Source: CAD feature listing. Evaluate the final solid. Frame: model axes, mm. A direction names the side the tool comes from. Give positions to 0.01 mm unless a question says otherwise; leave off trailing zeros. Loops run counter-clockwise (first coordinate to the right, second up) from the corner with the lowest first, then second, coordinate; pieces in that order, holes last. Notation, with made-up numbers: (27.25, -25.5) - (57.25, -25.5) arc R33 ccw to (57.25, 2.5) - close; hole circle Ø6 at (39, 72). An arc over 180 degrees is marked (long way). Put each result on its own line as item: value.
```python
from build123d import *

# Parameters (mm, degrees)
SKETCH1_R            = 14.2875
SKETCH1_R_2          = 2.54
BOSS_EXTRUDE1_DEPTH  = 3.175
CUT_EXTRUDE1_DEPTH   = 162.674043733
FILLET3_R            = 6.35
BOSS_EXTRUDE3_START  = -3.175
SKETCH3_R            = 2.54
BOSS_EXTRUDE3_DEPTH  = 3.175
SKETCH6_R            = 2.54
BOSS_EXTRUDE4_DEPTH  = 3.175
FILLET2_R            = 6.35
CUT_EXTRUDE2_DEPTH   = 168.423732074
CUT_EXTRUDE3_DEPTH   = 168.423732074
CUT_EXTRUDE4_DEPTH   = 168.265702461
BOSS_EXTRUDE8_START  = -3.175
SKETCH15_R           = 2.54
BOSS_EXTRUDE8_DEPTH  = 3.175
FILLET4_R            = 2.54
BOSS_EXTRUDE9_DEPTH  = 3.175
SKETCH17_R           = 14.2875
BOSS_EXTRUDE10_DEPTH = 3.175
CUT_EXTRUDE5_DEPTH   = 132.939082706
SKETCH20_R           = 14.2875
CUT_EXTRUDE6_DEPTH   = 132.939082706


with BuildPart() as part:
    # Sketch1 → Boss-Extrude1 (new body)
    with BuildSketch(Plane.XY):
        with BuildLine():
            Line((-8.89, 25.4), (8.89, 25.4))
            ThreePointArc((8.89, 25.4), (17.870256121, 21.680256121), (21.59, 12.7))
            Line((21.59, 12.7), (21.59, -117.775079775))
            ThreePointArc((21.59, -117.775079775), (21.127743647, -120.388718212), (19.797058824, -122.685251408))
            Line((19.797058824, -122.685251408), (-7.952696208, -155.616779465))
            ThreePointArc((-7.952696208, -155.616779465), (-12.268297602, -157.851943494), (-16.900388255, -156.380852124))
            Line((-16.900388255, -156.380852124), (-32.439211784, -143.287061102))
            ThreePointArc((-32.439211784, -143.287061102), (-34.674375812, -138.971459708), (-33.203284443, -134.339369055))
            Line((-33.203284443, -134.339369055), (-23.382941176, -122.685251408))
            ThreePointArc((-23.382941176, -122.685251408), (-22.052256353, -120.388718212), (-21.59, -117.775079775))
            Line((-21.59, -117.775079775), (-21.59, 12.7))
            ThreePointArc((-21.59, 12.7), (-17.870256121, 21.680256121), (-8.89, 25.4))
        make_face()
        Circle(SKETCH1_R, mode=Mode.SUBTRACT)
        with Locations((0, -101.6)):
            Circle(SKETCH1_R, mode=Mode.SUBTRACT)
        with Locations((-18.532085478, -142.550133084)):
            Circle(SKETCH1_R_2, mode=Mode.SUBTRACT)
        with Locations((0, -50.8)):
            Circle(SKETCH1_R_2, mode=Mode.SUBTRACT)
    extrude(amount=BOSS_EXTRUDE1_DEPTH)

    # Sketch2 → Cut-Extrude1 (cut, through all)
    with BuildSketch(Plane.XY):
        with BuildLine():
            ThreePointArc((19.159083004, -91.647229609), (9.182340769, -50.8), (19.159083004, -9.952770391))
            ThreePointArc((19.159083004, -9.952770391), (20.973467787, -5.122670102), (21.59, 0))
            Line((21.59, 0), (27.94, 0))
            Line((27.94, 0), (27.94, -121.656687185))
            Line((27.94, -121.656687185), (-7.789552878, -164.05809836))
            Line((-7.789552878, -164.05809836), (-17.501317584, -155.874478972))
            Line((-17.501317584, -155.874478972), (16.51, -115.512152961))
            ThreePointArc((16.51, -115.512152961), (20.280273667, -109.005308906), (21.59, -101.6))
            ThreePointArc((21.59, -101.6), (20.973467787, -96.477329898), (19.159083004, -91.647229609))
        make_face()
        with BuildLine():
            Line((-21.59, -41.275), (-21.59, -60.325))
            ThreePointArc((-21.59, -60.325), (-12.065, -50.8), (-21.59, -41.275))
        make_face()
    extrude(amount=CUT_EXTRUDE1_DEPTH, mode=Mode.SUBTRACT)

    # Fillet3
    fillet3_edges = [part.edges().sort_by_distance(p)[0] for p in [
        (-21.59, -41.275, 1.5875),
        (-21.59, -60.325, 1.5875),
    ]]
    fillet(fillet3_edges, radius=FILLET3_R)

    # Sketch3 → Boss-Extrude3 (add)
    with BuildSketch(Plane.XY.offset(3.175).offset(BOSS_EXTRUDE3_START)):
        with BuildLine():
            Line((-27.351416194, -127.394768527), (-36.025496499, -137.688579))
            ThreePointArc((-36.025496499, -137.688579), (-37.217489152, -141.441859142), (-35.4063854, -144.93869507))
            Line((-35.4063854, -144.93869507), (-24.403104784, -154.210610454))
            ThreePointArc((-24.403104784, -154.210610454), (-19.771014132, -155.681701823), (-15.455412737, -153.446537795))
            Line((-15.455412737, -153.446537795), (-7.557639641, -144.073996091))
            Line((-7.557639641, -144.073996091), (-27.351416194, -127.394768527))
        make_face()
        with Locations((-18.532085478, -142.550133084)):
            Circle(SKETCH3_R, mode=Mode.SUBTRACT)
    extrude(amount=BOSS_EXTRUDE3_DEPTH)

    # Sketch6 → Boss-Extrude4 (add)
    with BuildSketch(Plane.XY.offset(3.175)):
        Polygon((-35.4063854, -144.93869507), (-63.620410749, -121.164144113), (-51.344981666, -106.596497054), (-27.065569901, -127.055545526), align=None)
        with Locations((-52.626813855, -117.972130278)):
            Circle(SKETCH6_R, mode=Mode.SUBTRACT)
    extrude(amount=-BOSS_EXTRUDE4_DEPTH)

    # Fillet2
    fillet2_edges = [part.edges().sort_by_distance(p)[0] for p in [
        (-63.620410749, -121.164144113, 1.5875),
        (-51.344981666, -106.596497054, 1.5875),
        (-27.065569901, -127.055545526, 1.5875),
    ]]
    fillet(fillet2_edges, radius=FILLET2_R)

    # Sketch7 → Cut-Extrude2 (cut, through all)
    with BuildSketch(Plane.XY.offset(3.175)):
        with BuildLine():
            Line((-21.59, 0), (-21.59, 31.75))
            Line((-21.59, 31.75), (21.59, 31.75))
            Line((21.59, 31.75), (21.59, 0))
            ThreePointArc((21.59, 0), (0, 21.59), (-21.59, 0))
        make_face()
    extrude(amount=-CUT_EXTRUDE2_DEPTH, mode=Mode.SUBTRACT)

    # Sketch10 → Cut-Extrude3 (cut, through all)
    with BuildSketch(Plane.XY.offset(3.175)):
        with BuildLine():
            Line((-18.151882461, -155.32628042), (-17.361482582, -157.512020269))
            Line((-17.361482582, -157.512020269), (-14.375706423, -156.432313955))
            Line((-14.375706423, -156.432313955), (-15.455412737, -153.446537795))
            ThreePointArc((-15.455412737, -153.446537795), (-16.679911193, -154.563907595), (-18.151882461, -155.32628042))
        make_face()
    extrude(amount=-CUT_EXTRUDE3_DEPTH, mode=Mode.SUBTRACT)

    # Sketch12 → Cut-Extrude4 (cut, through all)
    with BuildSketch(Plane.XY.offset(3.175)):
        with BuildLine():
            Line((-21.59, -101.6), (-72.39, -101.6))
            Line((-72.39, -101.6), (-72.39, -165.1))
            Line((-72.39, -165.1), (16.51, -165.1))
            Line((16.51, -165.1), (16.51, -115.512152961))
            ThreePointArc((16.51, -115.512152961), (-7.405308906, -121.880273667), (-21.59, -101.6))
        make_face()
    extrude(amount=-CUT_EXTRUDE4_DEPTH, mode=Mode.SUBTRACT)

    # Sketch15 → Boss-Extrude8 (add)
    with BuildSketch(Plane.XY.offset(3.175).offset(BOSS_EXTRUDE8_START)):
        with BuildLine():
            ThreePointArc((-34.29, -3.81), (-30.887045256, -16.51), (-21.59, -25.807045256))
            Line((-21.59, -25.807045256), (-21.59, 0))
            ThreePointArc((-21.59, 0), (-15.266435406, 15.266435406), (0, 21.59))
            Line((0, 21.59), (-8.89, 21.59))
            ThreePointArc((-8.89, 21.59), (-26.850512242, 14.150512242), (-34.29, -3.81))
        make_face()
        with Locations((-24.765, -3.81)):
            Circle(SKETCH15_R, mode=Mode.SUBTRACT)
    extrude(amount=BOSS_EXTRUDE8_DEPTH)

    # Fillet4
    fillet4_edges = [part.edges().sort_by_distance(p)[0] for p in [
        (-21.59, -25.807045256, 1.5875),
    ]]
    fillet(fillet4_edges, radius=FILLET4_R)

    # Sketch16 → Boss-Extrude9 (add, through all)
    with BuildSketch(Plane.XY.offset(3.175)):
        with BuildLine():
            Line((-21.59, -101.6), (-21.59, -105.77576))
            ThreePointArc((-21.59, -105.77576), (0, -127.36576), (21.59, -105.77576))
            Line((21.59, -105.77576), (21.59, -101.6))
            Line((21.59, -101.6), (4.517920132, -121.700477095))
            Line((4.517920132, -121.700477095), (-1.489522905, -121.700477095))
            Line((-1.489522905, -121.700477095), (-21.59, -101.6))
        make_face()
    extrude(amount=-BOSS_EXTRUDE9_DEPTH)

    # Sketch17 → Boss-Extrude10 (add, through all)
    with BuildSketch(Plane.XY.offset(3.175)):
        with Locations((0, -101.6)):
            Circle(SKETCH17_R)
    extrude(amount=-BOSS_EXTRUDE10_DEPTH)

    # Sketch19 → Cut-Extrude5 (cut, through all)
    with BuildSketch(Plane.XY.offset(3.175)):
        with BuildLine():
            Line((19.159083004, -91.647229609), (21.59, -91.647229609))
            Line((21.59, -91.647229609), (21.59, -105.77576))
            ThreePointArc((21.59, -105.77576), (20.977838358, -98.607693167), (19.159083004, -91.647229609))
        make_face()
    extrude(amount=-CUT_EXTRUDE5_DEPTH, mode=Mode.SUBTRACT)

    # Sketch20 → Cut-Extrude6 (cut, through all)
    with BuildSketch(Plane.XY.offset(3.175)):
        with Locations((0, -105.77576)):
            Circle(SKETCH20_R)
    extrude(amount=-CUT_EXTRUDE6_DEPTH, mode=Mode.SUBTRACT)


solid = part.part
```
1) Material intervals for line 1 along Y through (x, z) = (1, 0.3); line 2 along Y through (x, z) = (-5, 1.8); line 3 along Y through (x, z) = (7, 1.7), sorted ascending. Write a range as [from, to].
Check result:
line 1: [-127.34, -120.03], [-91.52, -53.13], [-48.47, -14.25], [14.25, 21.57]
line 2: [-126.78, -119.16], [-92.39, -13.38], [13.38, 21.59]
line 3: [-126.2, -118.23], [-93.32, -12.46], [12.46, 20.42]
2) Section query D-D, the plane x = -26. Output: boundary loops of the cut face in (y, z) (3 decimals).
Check result:
outline: (-22.583, 0) - (-6.03, 0) - (-6.03, 3.175) - (-22.583, 3.175) - close; (-1.59, 0) - (14.963, 0) - (14.963, 3.175) - (-1.59, 3.175) - close
3) Mould query, pull axis Y, two halves, no side actions, for faces 6 (the cylindrical face through (-1.86, -91.61, 1.61)), 7 (the flat face through (-7, -35, 0)), 8 (the cylindrical face through (-0.47, -127.36, 1.61)). Classes: pulls with the +Y half, pulls with the -Y half, needs draft (parallel to the pull), parting line crosses it, or undercut.
Check result:
face 6: undercut
face 7: needs draft
face 8: pulls with the -Y half
4) Section query B-B, the plane z = 2.05. State how many separate pieces and enclosed holes the cut face has, plus the area to 3 significant figures.
Check result:
separate pieces: 1
enclosed holes: 4
area: 4,270 mm²
5) Pin query (flat end, axial travel): P1, Ø1.5, axis at y = -110.5, z = 1.5, coming from the +X side; P2, Ø8, axis at x = -24.765, y = -3.81, coming from the -Z side; P3, Ø1, axis at x = -13.5, z = 1, coming from the +Y side; P4, Ø1, axis at y = -32, z = 1.5, coming from the -X side. Return the tip coordinate at first contact, or that it passes through.
Check result:
P1: x = 21.22
P2: z = 0
P3: y = 21.26
P4: x = -21.59
6) Access query for faces 1 (the cylindrical face through (20.995, -98.707, 1.61)), 2 (the cylindrical face through (-20.58, -39.69, 1.61)), 3 (the flat face through (-7, -35, 3.175)), 4 (the cylindrical face through (-0.33, -48.28, 1.57)), 5 (the flat face through (-21.59, -85, 2)). Directions: +Z, -Z, +X, -X, +Y, -Y. A direction counts if a zero-diameter tool reaches every point of the face in a straight line with its end or side. Return the directions, or none.
Check result:
face 1: +Z, -Z, +X
face 2: +Z, -Z, -X
face 3: +Z, +X, -X, +Y, -Y
face 4: +Z, -Z
face 5: +Z, -Z, -X, -Y
7) Section query C-C, the plane x = -5.5. Output: boundary loops of the cut face in (y, z) (3 decimals).
Check result:
outline: (-126.653, 0) - (-118.962, 0) - (-118.962, 3.175) - (-126.653, 3.175) - close; (-92.589, 0) - (-13.186, 0) - (-13.186, 3.175) - (-92.589, 3.175) - close; (13.186, 0) - (21.59, 0) - (21.59, 3.175) - (13.186, 3.175) - close
8) Section query A-A, the plane y = -50.8. Output: boundary loops of the cut face in (x, z) (3 decimals).
Check result:
outline: (-12.065, 0) - (-2.54, 0) - (-2.54, 3.175) - (-12.065, 3.175) - close; (2.54, 0) - (9.182, 0) - (9.182, 3.175) - (2.54, 3.175) - close
